Drawing for the job (mm, zero at the part's lowest x, y, z). A direction names the side the tool comes from. Round coordinates to 2 decimals unless told otherwise and drop trailing zeros. Order: outer loops, then holes, each group sorted by start corner. A loop starts at its lowest first (then second) coordinate and runs counter-clockwise, first axis right, second up. Notation, with made-up numbers: (-13.5, -36) - (15.5, -36) arc R8 cw to (15.5, -31) - close; hole circle Ø9 at (59.5, -4.75). An arc over 180 degrees is marked (long way). Answer as a JSON object with one key per item and string values.
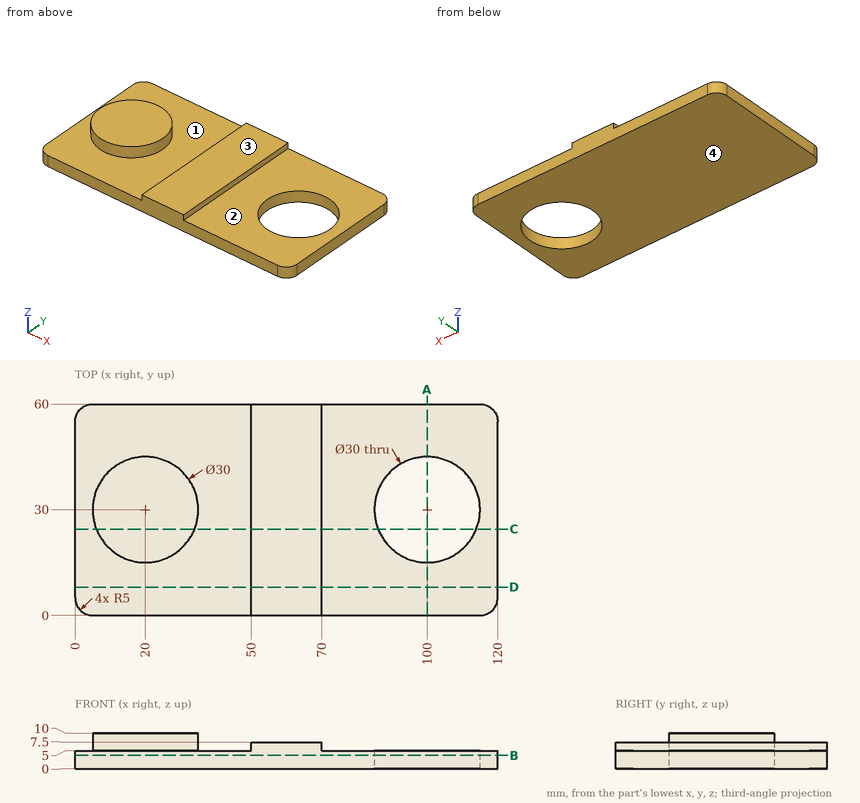
Item 1: Cut at A-A (x = 100). Write the cut outline in (y, z), plus the area to 3 significant figures.
Taken from the geometry:
{"outline": "(0, 0) - (15, 0) - (15, 5) - (0, 5) - close; (45, 0) - (60, 0) - (60, 5) - (45, 5) - close", "area": "150 mm2"}
Item 2: Probe L1, parallel to Y at x = 100, z = 3.35; L2, parallel to Z at x = 39, y = 51.5; L3, parallel to X at y = 40.5, z = 3.75. List the from-to ranges inside material, lowest first. Write a range as from..to.
Taken from the geometry:
{"L1": "0..15, 45..60", "L2": "0..5", "L3": "0..89.29, 110.71..120"}
Item 3: Drop flat-ended pins along their axis: P1, Ø2, axis at y = 27, z = 7, coming from the -X side; P2, Ø6, axis at x = 92.5, y = 20.5, coming from the +Z side; P3, Ø3, axis at x = 27, y = 11.5, coming from the -Z side; P4, Ø0.8, axis at y = 45, z = 6, coming from the +X side. Give the stop position or say it passes through.
Taken from the geometry:
{"P1": "x = 5.13", "P2": "z = 5", "P3": "z = 0", "P4": "x = 70"}
Item 4: Cut at C-C (y = 24.5). Write the cut outline in (x, z), plus the area to 3 significant figures.
Taken from the geometry:
{"outline": "(0, 0) - (86.04, 0) - (86.04, 5) - (70, 5) - (70, 7.5) - (50, 7.5) - (50, 5) - (33.96, 5) - (33.96, 10) - (6.04, 10) - (6.04, 5) - (0, 5) - close; (113.96, 0) - (120, 0) - (120, 5) - (113.96, 5) - close", "area": "650 mm2"}
Item 5: Cut at D-D (y = 8). Write the cut outline in (x, z).
Taken from the geometry:
{"outline": "(0, 0) - (120, 0) - (120, 5) - (70, 5) - (70, 7.5) - (50, 7.5) - (50, 5) - (0, 5) - close"}
Item 6: Two-plate mould, pull along X, no slides. Class the marked faces 1 and 2: pulls with the +X half, pulls with the -X half, needs draft (parallel to the pull), parting line crosses it, or undercut.
Taken from the geometry:
{"face 1": "undercut", "face 2": "needs draft"}
Item 7: Cut at B-B (z = 3.75). Write the cut outline in (x, y), plus the area to 3 significant figures.
Taken from the geometry:
{"outline": "(0, 5) arc R5 ccw to (5, 0) - (115, 0) arc R5 ccw to (120, 5) - (120, 55) arc R5 ccw to (115, 60) - (5, 60) arc R5 ccw to (0, 55) - close; hole circle Ø30 at (100, 30)", "area": "6,470 mm2"}
Item 8: Tool access for the marked faces 3 and 4: list every direction of +Z, -Z, +X, -X, +Y, -Y with a clear straight run to the whole face (end or side of a thin tool).
Taken from the geometry:
{"face 3": "+Z, +X, +Y, -Y", "face 4": "-Z, +X, -X, +Y, -Y"}
